```python
from build123d import *

# Parameters (mm, degrees)
BASPROSKE_W             = 5.5
BASPROSKE_H             = 44
TOOTHCUT_DEPTH          = 63.467991804
TEETHCUTS_COUNT         = 20
TEETHCUTS_ANGLE         = 342
BORSKE_R                = 0.5
BORE_DEPTH              = 50.0000508
CORTAR_EXTRUIR1_DEPTH   = 5.5
SALIENTE_EXTRUIR1_DEPTH = 5.5


with BuildPart() as part:
    # BasProSke → Base-Revolve (revolve)
    with BuildSketch(Plane(origin=(0, 0, 0), x_dir=(1, 0, 0), z_dir=(0, 1, 0)), mode=Mode.PRIVATE) as base_revolve_sk:
        with Locations((2.75, 22)):
            Rectangle(BASPROSKE_W, BASPROSKE_H)
    revolve(base_revolve_sk.sketch.rotate(Axis((-10, 0, 0), (1, 0, 0)), 180), axis=Axis((-10, 0, 0), (1, 0, 0)))

    # TooCutSke → ToothCut (cut, through all)
    with BuildSketch(Plane(origin=(0, 0, 0), x_dir=(0, 0, -1), z_dir=(1, 0, 0))):
        with BuildLine():
            ThreePointArc((1.961730392, 34.943978235), (0, 34.999), (-1.961730392, 34.943978235))
            ThreePointArc((-1.961730392, 34.943978235), (-3.235659864, 39.585086827), (-5.832115241, 43.637395396))
            ThreePointArc((-5.832115241, 43.637395396), (0, 44.0254), (5.832115241, 43.637395396))
            ThreePointArc((5.832115241, 43.637395396), (3.235659864, 39.585086827), (1.961730392, 34.943978235))
        make_face()
    toothcut = extrude(amount=TOOTHCUT_DEPTH, mode=Mode.SUBTRACT)

    # TeethCuts: ToothCut ×20 about axis
    teethcuts_axis = Axis((-10, 0, 0), (1, 0, 0))
    for i in range(1, TEETHCUTS_COUNT):
        add(toothcut.rotate(teethcuts_axis, i * TEETHCUTS_ANGLE / (TEETHCUTS_COUNT - 1)), mode=Mode.SUBTRACT)

    # BorSke → Bore (cut, symmetric)
    with BuildSketch(Plane(origin=(0, 0, 0), x_dir=(0, 0, -1), z_dir=(1, 0, 0))):
        with Locations(Location((0, 0, 0), (0, 0, 180))):
            Circle(BORSKE_R)
    extrude(amount=BORE_DEPTH, both=True, mode=Mode.SUBTRACT)

    # Croquis1 → Cortar-Extruir1 (cut)
    with BuildSketch(Plane(origin=(5.5, 0, 0), x_dir=(0, 0, -1), z_dir=(1, 0, 0))):
        with BuildLine():
            Line((-4, 0), (4, 0))
            ThreePointArc((4, 0), (0, -4), (-4, 0))
        make_face()
    extrude(amount=-CORTAR_EXTRUIR1_DEPTH, mode=Mode.SUBTRACT)

    # Croquis2 → Saliente-Extruir1 (add)
    with BuildSketch(Plane(origin=(5.5, 0, 0), x_dir=(0, 0, -1), z_dir=(1, 0, 0))):
        with BuildLine():
            Line((-0.5, 0), (0.5, 0))
            ThreePointArc((0.5, 0), (0, 0.5), (-0.5, 0))
        make_face()
    extrude(amount=-SALIENTE_EXTRUIR1_DEPTH)


solid = part.part
```
The model under review builds one solid part; all positions refer to its coordinate system, in mm. A direction names the side the tool comes from. Coordinates: 2 decimals unless noted, no trailing zeros. Write each loop counter-clockwise with the first axis right and the second up, starting at its lowest first coordinate (ties: lowest second). Pieces come first, ordered by that corner, then holes. Notation, with made-up numbers: (75.5, 83) - (87.5, 83) arc R33 ccw to (87.5, 112) - close; hole circle Ø2 at (-15, 63). An arc over 180 degrees is marked (long way). Answer in a Markdown table with one row per item. Add a question column.
Q1. To check wall thickness, follow line 1 along Z through (x, y) = (0.9, -39); line 2 along Y through (x, z) = (0.7, 28); line 3 along Z through (x, y) = (1.05, -1). State the ranges of each line that lie inside material, in increasing order. Write a range as from..to.
Q2. Consider section B-B on y = 11.5. Give the boundary of the cut face in (x, z).
Q3. For faces 1 (the face through (2.71, 9.15, -38.7)), 2 (the face through (2.712, 15.345, 36.686)), 3 (the face through (2.712, -39.633, 3.257)), list the 3-axis set-ups (+Z, -Z, +X, -X, +Y, -Y) from which the entire face can be reached by the end or side of a thin tool; tool diameter is ignored.
Q4. Clearance check with flat-ended pins moving along their axes: pin 1 (3 mm diameter, centred on x = 2, z = -3.5, fed in from -Y); pin 2 (1 mm diameter, centred on x = 1.5, y = 31, fed in from -Z). State where each tip first meets the part, or that it passes through.
Q5. Draft analysis for pull direction Z (two halves, no side actions). For faces 4 (the face through (3, 0, -35)), 5 (the face through (3, -28, 21)), 6 (the face through (2.712, 36.686, -15.345)), 7 (the face through (2.79, 39.21, 19.96)), state which applies: +Z half, -Z half, draft (parallel to the pull), parting line (faces both ways), or undercut.
Q6. Consider section A-A on z = 0. Give the boundary of the cut face in (x, y), then the cut area to 3 significant figures.
Q7. Consider section C-C on z = 25. Give the boundary of the cut face in (x, y), then the cut area to 3 significant figures.
Answers below:
| question | item | result |
|---|---|---|
| 1 | line 1 | -20.37..-17.95, -9.11..-2.99, 2.99..9.11, 17.95..20.37 |
| 1 | line 2 | -31.15..-23.01, -21..21, 23.01..31.15 |
| 1 | line 3 | -34.98..-3.87, 3.87..34.98 |
| 2 | outline | (0, -33.06) - (5.5, -33.06) - (5.5, 33.06) - (0, 33.06) - close |
| 3 | face 1 | +X, -X |
| 3 | face 2 | +Z, +X, -X |
| 3 | face 3 | +X, -X, -Y |
| 4 | pin 1 | y = -42.61 |
| 4 | pin 2 | z = -31.71 |
| 5 | face 4 | -Z half |
| 5 | face 5 | undercut |
| 5 | face 6 | undercut |
| 5 | face 7 | +Z half |
| 6 | outline | (0, -35) - (5.5, -35) - (5.5, -4) - (0, -4) - close; (0, 0) - (5.5, 0) - (5.5, 35) - (0, 35) - close |
| 6 | area | 363 mm² |
| 7 | outline | (0, -29.57) - (5.5, -29.57) - (5.5, 29.57) - (0, 29.57) - close |
| 7 | area | 325 mm² |
